Could you check a few things on this model? Use its own coordinates, in mm. A direction names the side the tool comes from. Give positions to 0.01 mm unless a question says otherwise; leave off trailing zeros. Write each loop counter-clockwise with the first axis right and the second up, starting at its lowest first coordinate (ties: lowest second). Pieces come first, ordered by that corner, then holes. Notation, with made-up numbers: (13, 8.25) - (34, 8.25) arc R25 cw to (34, 37.25) - close; hole circle Ø7 at (-30, 42). An arc over 180 degrees is marked (long way). Answer as CSV lines item,"result". Start each with the question number.
Q1. If I drill on line 1 along Y through (x, z) = (3, 0); line 2 along Z through (x, y) = (-10.5, 50.5); line 3 along Z through (x, y) = (0.45, 41.47), over which ranges is the centre line in solid material (lowest first)?
Q2. Imagine slicing it at A-A on y = 41.47. List the corners of the cut face in (x, z) for me, and give its area (3 significant figures).
Q3. On a 3-axis mill with a long thin cutter (end or side, diameter ignored), from which of +Z, -Z, +X, -X, +Y, -Y can I reach the whole of each face in a straight line? I mean faces 1 (the face through (-0.127, 40, 9)), 2 (the face through (3.7, 52.85, 29.46)), 3 (the face through (1.2, 31.8, -32.9)). Say none if no direction works.
Q4. Imagine slicing it at B-B on x = -10.5. List the corners of the cut face in (y, z) for me, and give its area (3 significant figures).
Q5. Will these pins go through, and if not, where does the flat tip stop? pin 1 Ø0.9 at (x, z) = (16.5, 19) entering from +Y; pin 2 Ø0.8 at (x, y) = (10.5, 82) entering from +Z (3 decimals); pin 3 Ø10.5 at (y, z) = (77.98, 0) entering from +X.
Q6. Imagine slicing it at D-D on x = 3.5. List the corners of the cut face in (y, z) for me, and give its area (3 significant figures).
Q7. Imagine slicing it at C-C on z = -11.5. List the corners of the cut face in (x, y) for me.
Q8. We'd pull the mould along Y, two halves only. Please class faces 4 (the face through (1.161, 56.878, 34.845)), 5 (the face through (0, 0, 0)), 6 (the face through (-7, 20.32, -1)), 7 (the face through (15, 82, 10.16)): pulls with the +Y half, pulls with the -Y half, needs draft (parallel to the pull), parting line crosses it, or undercut.
```python
from build123d import *

# Parameters (mm, degrees)
SKETCH3_R                      = 4.953
POST_DEPTH                     = 13.97
SKETCH4_W                      = 24.13
SKETCH4_H                      = 85.725
BASE_DEPTH                     = 6.35
SKETCH5_W                      = 24.13
SKETCH5_H                      = 85.725
SKETCH5_W_2                    = 15.24
SKETCH5_H_2                    = 73.025
CAVITY_DEPTH                   = 69.85
MOTORHOLES_REACH               = 104.714
SKETCH8_R                      = 6.35
SKETCH8_R_2                    = 2.54
POWERSCREWHOLES_REACH          = 104.714
SKETCH7_R                      = 4.064
NUT_SOCKET_DEPTH               = 2.54
SKETCH12_W                     = 9.525
SKETCH12_H                     = 2.54
LIMITSWITCHSUPPORT_DEPTH       = 19.939
SKETCH20_R                     = 1.016
BOSS_EXTRUDE3_DEPTH            = 6.096
ZIPTIECUTOUT_REACH             = 106.211
SKETCH22_W                     = 3.81
SKETCH22_H                     = 1.524
ZIPTIECUTOUT_DIRECTION_2_REACH = 106.211


with BuildPart() as part:
    # Sketch3 → Post (new body)
    with BuildSketch(Plane(origin=(0, 0, 0), x_dir=(1, 0, 0), z_dir=(0, 1, 0))):
        with Locations(Location((0, 0, 0), (0, 0, 270))):
            Circle(SKETCH3_R)
    extrude(amount=POST_DEPTH)

    # Sketch4 → Base (add)
    with BuildSketch(Plane(origin=(0, 13.97, 0), x_dir=(1, 0, 0), z_dir=(0, 1, 0))):
        with Locations((-7.112, 0)):
            Rectangle(SKETCH4_W, SKETCH4_H)
    extrude(amount=BASE_DEPTH)

    # Sketch5 → Cavity (add)
    with BuildSketch(Plane(origin=(0, 20.32, 0), x_dir=(1, 0, 0), z_dir=(0, 1, 0))):
        with Locations((-7.112, 0)):
            Rectangle(SKETCH5_W, SKETCH5_H)
        with Locations((-5.207, 0)):
            Rectangle(SKETCH5_W_2, SKETCH5_H_2, mode=Mode.SUBTRACT)
    extrude(amount=CAVITY_DEPTH)

    # Sketch8 → MotorHoles (cut, up to next)
    with BuildSketch(Plane(origin=(4.953, 0, 0), x_dir=(0, 0, -1), z_dir=(1, 0, 0)), mode=Mode.PRIVATE) as motorholes_sk1:
        with Locations((0, 41.47)):
            Circle(SKETCH8_R)
    motorholes_tool1 = extrude(motorholes_sk1.sketch, amount=-MOTORHOLES_REACH, mode=Mode.PRIVATE) & part.part
    # Sketch8 → MotorHoles (cut, up to next)
    with BuildSketch(Plane(origin=(4.953, 0, 0), x_dir=(0, 0, -1), z_dir=(1, 0, 0)), mode=Mode.PRIVATE) as motorholes_sk2:
        with Locations((-30.629352104, 55.107066169)):
            Circle(SKETCH8_R_2)
    motorholes_tool2 = extrude(motorholes_sk2.sketch, amount=-MOTORHOLES_REACH, mode=Mode.PRIVATE) & part.part
    # Sketch8 → MotorHoles (cut, up to next)
    with BuildSketch(Plane(origin=(4.953, 0, 0), x_dir=(0, 0, -1), z_dir=(1, 0, 0)), mode=Mode.PRIVATE) as motorholes_sk3:
        with Locations((30.629352104, 27.832933831)):
            Circle(SKETCH8_R_2)
    motorholes_tool3 = extrude(motorholes_sk3.sketch, amount=-MOTORHOLES_REACH, mode=Mode.PRIVATE) & part.part
    add(motorholes_tool1.solids().sort_by_distance((4.953, 41.47, 0))[0], mode=Mode.SUBTRACT)
    add(motorholes_tool2.solids().sort_by_distance((4.953, 55.107066, 30.629352))[0], mode=Mode.SUBTRACT)
    add(motorholes_tool3.solids().sort_by_distance((4.953, 27.832934, -30.629352))[0], mode=Mode.SUBTRACT)

    # PowerscrewHoles: up to this face of the body (flat: up to its plane)
    powerscrewholes_end = Plane(part.part.faces().sort_by_distance((-19.177, 52.07, 0))[0])
    # Sketch7 → PowerscrewHoles (cut, up to the picked face)
    with BuildSketch(Plane(origin=(4.953, 0, 0), x_dir=(0, 0, -1), z_dir=(1, 0, 0)), mode=Mode.PRIVATE) as powerscrewholes_sk1:
        with Locations((0, 77.9825)):
            Circle(SKETCH7_R)
    powerscrewholes_tool1 = split(extrude(powerscrewholes_sk1.sketch, amount=-POWERSCREWHOLES_REACH, mode=Mode.PRIVATE), bisect_by=powerscrewholes_end, keep=Keep.BOTH, mode=Mode.PRIVATE)
    add(powerscrewholes_tool1.solids().sort_by(Axis((4.953, 77.9825, 0), (-1, 0, 0)))[0], mode=Mode.SUBTRACT)

    # Sketch10 → Nut Socket (add)
    with BuildSketch(Plane.ZY.offset(-2.413)):
        with BuildLine():
            Line((-36.5125, 90.17), (-30.688519739, 90.17))
            ThreePointArc((-30.688519739, 90.17), (-28.656384533, 61.577256158), (-5.028558234, 45.347641304))
            ThreePointArc((-5.028558234, 45.347641304), (0, 35.12), (5.028558234, 45.347641304))
            ThreePointArc((5.028558234, 45.347641304), (28.656384533, 61.577256158), (30.688519739, 90.17))
            Line((30.688519739, 90.17), (36.5125, 90.17))
            Line((36.5125, 90.17), (36.5125, 20.32))
            Line((36.5125, 20.32), (-36.5125, 20.32))
            Line((-36.5125, 20.32), (-36.5125, 90.17))
        make_face()
        Polygon((-26.057352104, 30.472579262), (-30.629352104, 33.112224692), (-35.201352104, 30.472579262), (-35.201352104, 25.1932884), (-30.629352104, 22.553642969), (-26.057352104, 25.1932884), align=None, mode=Mode.SUBTRACT)
        Polygon((32.712972872, 50.256351119), (35.872004948, 54.486177161), (33.788384179, 59.336892211), (28.545731335, 59.957781219), (25.38669926, 55.727955177), (27.470320028, 50.877240127), align=None, mode=Mode.SUBTRACT)
    extrude(amount=NUT_SOCKET_DEPTH)

    # Sketch12 → LimitSwitchSupport (add)
    with BuildSketch(Plane(origin=(4.953, 0, 0), x_dir=(0, 0, -1), z_dir=(1, 0, 0))):
        with Locations((-14.9225, 82.3005)):
            Rectangle(SKETCH12_W, SKETCH12_H)
    extrude(amount=LIMITSWITCHSUPPORT_DEPTH)

    # Rib2: read off the stored shape, not the designer's step
    # Rib2: loft between two sections, ruled curve by curve
    rib2_from = [
        Edge.make_line((14.478, 90.17, 13.6525), (14.478, 90.17, 16.1925)),
        Edge.make_line((4.953, 90.17, 16.1925), (14.478, 90.17, 16.1925)),
        Edge.make_line((4.953, 90.17, 13.6525), (14.478, 90.17, 13.6525)),
        Edge.make_line((4.953, 90.17, 13.6525), (4.953, 90.17, 16.1925)),
    ]
    rib2_to = [
        Edge.make_line((24.892, 83.5705, 11.884169305), (24.892, 83.5705, 17.960830695)),
        Edge.make_line((4.953, 83.5705, 17.960830695), (24.892, 83.5705, 17.960830695)),
        Edge.make_line((4.953, 83.5705, 11.884169305), (24.892, 83.5705, 11.884169305)),
        Edge.make_line((4.953, 83.5705, 11.884169305), (4.953, 83.5705, 17.960830695)),
    ]
    rib2 = Solid(Shell([*[Face.make_surface_from_curves(rib2_from[k], rib2_to[k]) for k in range(4)], Face(Wire(rib2_from)), Face(Wire(rib2_to))]))
    add(rib2)

    # Sketch20 → Boss-Extrude3 (add)
    with BuildSketch(Plane.XZ.offset(-81.0305)):
        with Locations(Location((9.906, 17.399, 0), (0, 0, 90))):
            Circle(SKETCH20_R)
        with Locations(Location((19.939, 17.399, 0), (0, 0, 90))):
            Circle(SKETCH20_R)
    extrude(amount=BOSS_EXTRUDE3_DEPTH)

    # ZipTieCutout: up to this plane
    ziptiecutout_end = Plane(origin=(2.8575, 90.17, 13.6525), z_dir=(0, -0.25881904510252135, 0.9659258262890681))
    # Sketch22 → ZipTieCutout (cut, up to the surface)
    with BuildSketch(Plane(origin=(0, 7.096196959, 14.9225), x_dir=(0.9999812488409504, 0.00612388491835337, 0), z_dir=(0, 0, 1)), mode=Mode.PRIVATE) as ziptiecutout_sk1:
        with Locations((10.192898839, 77.16364952)):
            Rectangle(SKETCH22_W, SKETCH22_H)
    ziptiecutout_tool1 = split(extrude(ziptiecutout_sk1.sketch, amount=-ZIPTIECUTOUT_REACH, mode=Mode.PRIVATE), bisect_by=ziptiecutout_end, keep=Keep.BOTH, mode=Mode.PRIVATE)
    add(ziptiecutout_tool1.solids().sort_by_distance((9.720166, 84.32082, 14.9225))[0], mode=Mode.SUBTRACT)

    # ZipTieCutout direction 2: up to this plane
    ziptiecutout_direction_2_end = Plane(origin=(2.8575, 90.17, 16.1925), z_dir=(0, 0.25881904510252135, 0.9659258262890681))
    # Sketch22 → ZipTieCutout direction 2 (cut, up to the surface)
    with BuildSketch(Plane(origin=(0, 7.096196959, 14.9225), x_dir=(0.9999812488409504, 0.00612388491835337, 0), z_dir=(0, 0, 1)), mode=Mode.PRIVATE) as ziptiecutout_direction_2_sk1:
        with Locations((10.192898839, 77.16364952)):
            Rectangle(SKETCH22_W, SKETCH22_H)
    ziptiecutout_direction_2_tool1 = split(extrude(ziptiecutout_direction_2_sk1.sketch, amount=ZIPTIECUTOUT_DIRECTION_2_REACH, mode=Mode.PRIVATE), bisect_by=ziptiecutout_direction_2_end, keep=Keep.BOTH, mode=Mode.PRIVATE)
    add(ziptiecutout_direction_2_tool1.solids().sort_by_distance((9.720166, 84.32082, 14.9225))[0], mode=Mode.SUBTRACT)


solid = part.part
```
Conclusion:
1,line 1,"0 to 35.12, 47.82 to 73.92, 82.05 to 90.17"
1,line 2,"-42.86 to -36.51, 36.51 to 42.86"
1,line 3,"-42.86 to -6.35, 6.35 to 42.86"
2,outline,"(-19.18, -42.86) - (4.95, -42.86) - (4.95, -6.35) - (-0.13, -6.35) - (-0.13, -36.51) - (-12.83, -36.51) - (-12.83, 36.51) - (-0.13, 36.51) - (-0.13, 6.35) - (4.95, 6.35) - (4.95, 42.86) - (-19.18, 42.86) - close"
2,area,"1,080 mm^2"
3,face 1,"+Y"
3,face 2,"+X"
3,face 3,"none"
4,outline,"(13.97, -42.86) - (90.17, -42.86) - (90.17, -36.51) - (20.32, -36.51) - (20.32, 36.51) - (90.17, 36.51) - (90.17, 42.86) - (13.97, 42.86) - close"
4,area,"1,430 mm^2"
5,pin 1,"y = 83.57"
5,pin 2,"z = 19.685"
5,pin 3,"x = 4.95"
6,outline,"(0, -3.5) - (13.97, -3.5) - (13.97, -42.86) - (90.17, -42.86) - (90.17, 42.86) - (13.97, 42.86) - (13.97, 3.5) - (0, 3.5) - close; hole circle Ø5.08 at (27.83, -30.63); hole circle Ø12.7 at (41.47, 0); hole circle Ø5.08 at (55.11, 30.63); hole circle Ø8.13 at (77.98, 0)"
6,area,"6,410 mm^2"
7,outline,"(-19.18, 13.97) - (4.95, 13.97) - (4.95, 90.17) - (2.41, 90.17) - (2.41, 47.03) - (-0.13, 47.03) - (-0.13, 20.32) - (-12.83, 20.32) - (-12.83, 90.17) - (-19.18, 90.17) - close"
8,face 4,"undercut"
8,face 5,"pulls with the -Y half"
8,face 6,"pulls with the +Y half"
8,face 7,"needs draft"
